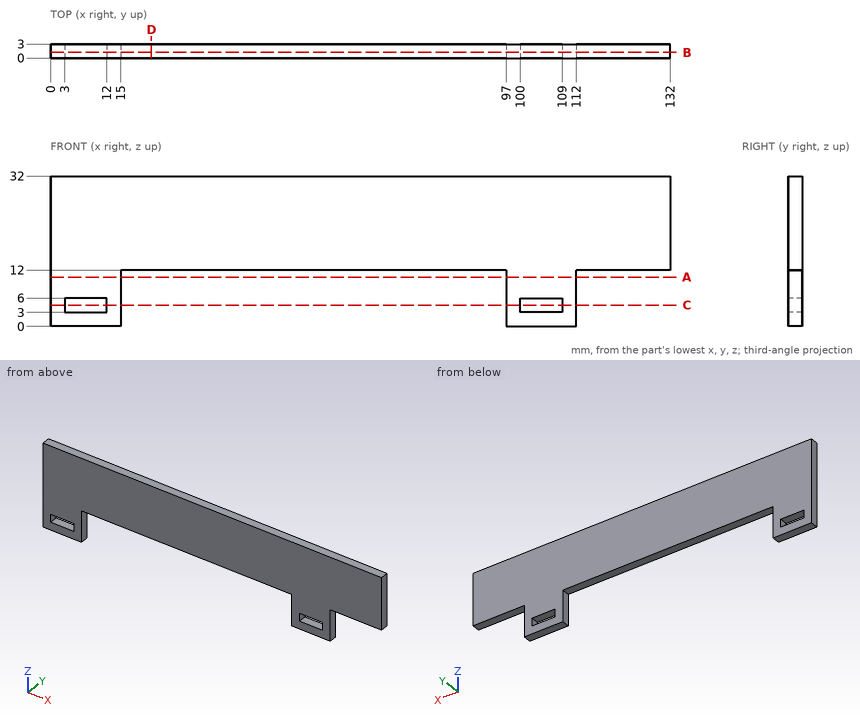
Design review of the part shown in the three views and the two pictorial views. Dimensions are in mm from the part's minimum x, y and z. Coordinates: 2 decimals unless noted, no trailing zeros. Order: outer loops, then holes, each group sorted by start corner. A loop starts at its lowest first (then second) coordinate and runs counter-clockwise, first axis right, second up.
Item 1: Take a section at D-D, the plane x = 21.5. Write out the cut boundary in (y, z), then the cut area to 3 significant figures.
Item 2: For line 1 (X direction, y = 1.85, z = 5.5); line 2 (Z direction, x = 6, y = 2.5); line 3 (X direction, y = 0.85, z = 9), list the stretches that pass through material, from the lowest coordinate up.
Item 3: Take a section at B-B, the plane y = 1.2. Write out the cut boundary in (x, z), then the cut area to 3 significant figures.
Item 4: For pin 1 Ø1 at (x, z) = (36, 11) entering from -Y; pin 2 Ø8 at (x, z) = (66, 8.5) entering from -Y; pin 3 Ø1.5 at (y, z) = (2, 5) entering from +X, all flat-tipped, find the tip position at first contact; note any pin that passes through.
Item 5: Take a section at A-A, the plane z = 10.5. Write out the cut boundary in (x, y), then the cut area to 3 significant figures.
Item 6: Take a section at C-C, the plane z = 4.5. Write out the cut boundary in (x, y).
The answers:
1. outline: (0, 12) - (3, 12) - (3, 32) - (0, 32) - close
1. area: 60.0 mm2
2. line 1: x = 0 to 3, 12 to 15, 97 to 100, 109 to 112
2. line 2: z = 0 to 3, 6 to 32
2. line 3: x = 0 to 15, 97 to 112
3. outline: (0, 0) - (15, 0) - (15, 12) - (97, 12) - (97, 0) - (112, 0) - (112, 12) - (132, 12) - (132, 32) - (0, 32) - close; hole (3, 3) - (12, 3) - (12, 6) - (3, 6) - close; hole (100, 3) - (109, 3) - (109, 6) - (100, 6) - close
3. area: 2,950 mm2
4. pin 1: passes through
4. pin 2: stops at y = 0
4. pin 3: stops at x = 112
5. outline: (0, 0) - (15, 0) - (15, 3) - (0, 3) - close; (97, 0) - (112, 0) - (112, 3) - (97, 3) - close
5. area: 90.0 mm2
6. outline: (0, 0) - (3, 0) - (3, 3) - (0, 3) - close; (12, 0) - (15, 0) - (15, 3) - (12, 3) - close; (97, 0) - (100, 0) - (100, 3) - (97, 3) - close; (109, 0) - (112, 0) - (112, 3) - (109, 3) - close
